Verification items for the finished model (mm, model axes). A direction names the side the tool comes from. Give positions to 0.01 mm unless a question says otherwise; leave off trailing zeros. Loops run counter-clockwise (first coordinate to the right, second up) from the corner with the lowest first, then second, coordinate; pieces in that order, holes last. Notation, with made-up numbers: M -39,33 L -30,33 A5 cw -30,38 Z; hole C 0.25,-33 d11. An arc over 180 degrees is marked long. Use a Markdown table: item, result.
from build123d import *

# Parameters (mm, degrees)
SKETCH1_W           = 25.4
SKETCH1_H           = 25.4
BOSS_EXTRUDE1_DEPTH = 12.7
SKETCH2_R           = 2.286
BOSS_EXTRUDE2_DEPTH = 3.175


with BuildPart() as part:
    # Sketch1 → Boss-Extrude1 (new body, symmetric)
    with BuildSketch(Plane(origin=(0, 0, 0), x_dir=(1, 0, 0), z_dir=(0, 1, 0))):
        Rectangle(SKETCH1_W, SKETCH1_H)
    extrude(amount=BOSS_EXTRUDE1_DEPTH, both=True)

    # Sketch2 → Boss-Extrude2 (add)
    with BuildSketch(Plane(origin=(0, 12.7, 0), x_dir=(1, 0, 0), z_dir=(0, 1, 0))):
        Circle(SKETCH2_R)
    extrude(amount=BOSS_EXTRUDE2_DEPTH)


solid = part.part
(1) Gauge pin test, flat end, axial feed: P1, Ø10, axis at x = 9.5, z = -6, coming from the +Y side. Record the tip position at first contact, or that the pin passes through.
Results below:
| item | result |
|---|---|
| P1 | y = 12.7 |
(2) Cross-section at B-B on z = 0. Record the cut outline in (x, y) (3 decimals), then the cut area to 3 significant figures.
Results below:
| item | result |
|---|---|
| outline | M -12.7,-12.7 L 12.7,-12.7 L 12.7,12.7 L 2.286,12.7 L 2.286,15.875 L -2.286,15.875 L -2.286,12.7 L -12.7,12.7 Z |
| area | 660 mm^2 |
(3) Material ranges on line 1 (Y direction, x = -0.75, z = -10); line 2 (X direction, y = 14, z = -0.75), recorded low to high.
Results below:
| item | result |
|---|---|
| line 1 | -12.7 to 12.7 |
| line 2 | -2.16 to 2.16 |
(4) Cross-section at C-C on z = 6. Record the cut outline in (x, y), then the cut area to 3 significant figures.
Results below:
| item | result |
|---|---|
| outline | M -12.7,-12.7 L 12.7,-12.7 L 12.7,12.7 L -12.7,12.7 Z |
| area | 645 mm^2 |
(5) Set-up check for faces 1 (the cylindrical face through (-0.5, 14.27, 2.23)), 2 (the flat face through (12.7, 0, 0)): record each of +Z, -Z, +X, -X, +Y, -Y from which the full face is reachable in a straight line by a thin tool's end or side.
Results below:
| item | result |
|---|---|
| face 1 | +Y |
| face 2 | +Z, -Z, +X, +Y, -Y |
(6) Cross-section at A-A on x = 0. Record the cut outline in (y, z) (3 decimals).
Results below:
| item | result |
|---|---|
| outline | M -12.7,-12.7 L 12.7,-12.7 L 12.7,-2.286 L 15.875,-2.286 L 15.875,2.286 L 12.7,2.286 L 12.7,12.7 L -12.7,12.7 Z |
